from build123d import *

# Parameters (mm, degrees)
SKETCH1_W           = 254
SKETCH1_H           = 254
BOSS_EXTRUDE1_DEPTH = 3.175
SKETCH2_R           = 3.175
SKETCH2_W           = 25.4
SKETCH2_H           = 25.4
CUT_EXTRUDE1_DEPTH  = 4.175
FILLET1_R           = 152.4
FILLET2_R           = 76.2


with BuildPart() as part:
    # Sketch1 → Boss-Extrude1 (new body)
    with BuildSketch(Plane(origin=(0, 0, 0), x_dir=(0, 0, -1), z_dir=(1, 0, 0))):
        with Locations((127, 127)):
            Rectangle(SKETCH1_W, SKETCH1_H)
    extrude(amount=BOSS_EXTRUDE1_DEPTH)

    # Sketch2 → Cut-Extrude1 (cut, through all)
    with BuildSketch(Plane(origin=(3.175, 0, 0), x_dir=(0, 0, -1), z_dir=(1, 0, 0))):
        with Locations((102.775, 52.775)):
            Circle(SKETCH2_R)
        with Locations((96.425, 165.10000014)):
            Circle(SKETCH2_R)
        with Locations((45.625, 198.825)):
            Circle(SKETCH2_R)
        with Locations((12.7, 165.1)):
            Circle(SKETCH2_R)
        with Locations((12.7, 241.3)):
            Circle(SKETCH2_R)
        with Locations((12.7, 12.7)):
            Circle(SKETCH2_R)
        with Locations((241.3, 165.1)):
            Circle(SKETCH2_R)
        with Locations((12.7, 82.55)):
            Rectangle(SKETCH2_W, SKETCH2_H)
    extrude(amount=-CUT_EXTRUDE1_DEPTH, mode=Mode.SUBTRACT)

    # Fillet1
    fillet1_edges = [part.edges().sort_by_distance(p)[0] for p in [
        (1.5875, 0, -254),
    ]]
    fillet(fillet1_edges, radius=FILLET1_R)

    # Fillet2
    fillet2_edges = [part.edges().sort_by_distance(p)[0] for p in [
        (1.5875, 254, -254),
    ]]
    fillet(fillet2_edges, radius=FILLET2_R)


solid = part.part
Geometry: final body of the model. Coordinates: model frame, mm. Give positions to 0.01 mm unless a question says otherwise; leave off trailing zeros. Write each loop counter-clockwise with the first axis right and the second up, starting at its lowest first coordinate (ties: lowest second). Pieces come first, ordered by that corner, then holes.
(1) Cut plane A-A, the plane y = 165.1. Return loops of the section in (x, z) (3 decimals), then the cut area to 3 significant figures.
(2) First-contact query: P1, Ø5, axis at y = 165.1, z = -12.7, coming from the +X side; P2, Ø1, axis at x = 1, y = 85.5, coming from the +Z side. Flat tips, straight axial feed; report the tip coordinate or a pass-through.
(3) Cut plane D-D, the plane z = -188. Return loops of the section in (x, y) (3 decimals).
(4) Cut plane C-C, the plane x = 2.3. Return loops of the section in (y, z) (3 decimals), then the cut area to 3 significant figures.
(5) Cut plane B-B, the plane y = 12.7. Return loops of the section in (x, z) (3 decimals), then the cut area to 3 significant figures.
(6) Mould query, pull axis Y, two halves, no side actions, for faces 1 (the flat face through (0, 129, -125)), 2 (the cylindrical face through (1.61, 231.086, -232.271)), 3 (the cylindrical face through (1.61, 162, -12.01)), 4 (the cylindrical face through (1.61, 43.459, -208.172)). Classes: released by +Y, released by -Y, zero draft, split by the parting line, or undercut.
(7) Ray query, line 1 (Y direction, x = 1.5, z = -12.7) (3 decimals); line 2 (Y direction, x = 2, z = -17); line 3 (Z direction, x = 3, y = 133). Return the intervals inside material, ascending.
Values follow:
1. outline: (0, -254) - (3.175, -254) - (3.175, -244.475) - (0, -244.475) - close; (0, -238.125) - (3.175, -238.125) - (3.175, -99.6) - (0, -99.6) - close; (0, -93.25) - (3.175, -93.25) - (3.175, -15.875) - (0, -15.875) - close; (0, -9.525) - (3.175, -9.525) - (3.175, 0) - (0, 0) - close
1. area: 746 mm2
2. P1: passes through
2. P2: stops at z = -25.4
3. outline: (0, 26.858) - (3.175, 26.858) - (3.175, 253.314) - (0, 253.314) - close
4. outline: (0, -101.6) arc R152.4 ccw to (152.4, -254) - (177.8, -254) arc R76.2 ccw to (254, -177.8) - (254, 0) - (95.25, 0) - (95.25, -25.4) - (69.85, -25.4) - (69.85, 0) - (0, 0) - close; hole circle Ø6.35 at (12.7, -12.7); hole circle Ø6.35 at (52.775, -102.775); hole circle Ø6.35 at (165.1, -241.3); hole circle Ø6.35 at (165.1, -96.425); hole circle Ø6.35 at (165.1, -12.7); hole circle Ø6.35 at (198.825, -45.625); hole circle Ø6.35 at (241.3, -12.7)
4. area: 57,400 mm2
5. outline: (0, -162.507) - (3.175, -162.507) - (3.175, -15.875) - (0, -15.875) - close; (0, -9.525) - (3.175, -9.525) - (3.175, 0) - (0, 0) - close
5. area: 496 mm2
6. face 1: zero draft
6. face 2: released by +Y
6. face 3: undercut
6. face 4: released by -Y
7. line 1: y = 0 to 9.525, 15.875 to 69.85, 95.25 to 161.925, 168.275 to 238.125, 244.475 to 254
7. line 2: y = 0 to 69.85, 95.25 to 254
7. line 3: z = -252.76 to 0
